Design review of the part built by this model. Coordinates are the model's own, in mm. Face numbers are marked on the shaded views. A direction names the side the tool comes from. Give positions to 0.01 mm unless a question says otherwise; leave off trailing zeros. Write each loop counter-clockwise with the first axis right and the second up, starting at its lowest first coordinate (ties: lowest second). Pieces come first, ordered by that corner, then holes.
```python
from build123d import *

# Parameters (mm, degrees)
F0_R     = 14.85
F0_R_2   = 2.25
F1_DEPTH = 13
F2_R     = 15.05
F3_DEPTH = 6
F4_R     = 14.6
F4_R_2   = 2.25
F5_DEPTH = 6.8
F6_R     = 2


with BuildPart() as f1:
    # F0 (on Top) → F1 (new body)
    with BuildSketch(Plane.XY):
        with BuildLine():
            ThreePointArc((10.083278, -13.5), (15.063627, -7.550472), (16.85, 0))
            ThreePointArc((16.85, 0), (15.063627, 7.550472), (10.083278, 13.5))
            ThreePointArc((10.083278, 13.5), (0, 16.85), (-10.083278, 13.5))
            ThreePointArc((-10.083278, 13.5), (-16.85, 0), (-10.083278, -13.5))
            ThreePointArc((-10.083278, -13.5), (0, -16.85), (10.083278, -13.5))
        make_face()
        Circle(F0_R, mode=Mode.SUBTRACT)
        with BuildLine():
            ThreePointArc((10.083278, 13.5), (15.063627, 7.550472), (16.85, 0))
            ThreePointArc((16.85, 0), (15.063627, -7.550472), (10.083278, -13.5))
            Line((10.083278, -13.5), (29.177113, -5.759277))
            ThreePointArc((29.177113, -5.759277), (30.538106, -4.655164), (31.05, -2.979058))
            Line((31.05, -2.979058), (31.05, 0))
            Line((31.05, 0), (31.05, 2.979058))
            ThreePointArc((31.05, 2.979058), (30.538106, 4.655164), (29.177113, 5.759277))
            Line((29.177113, 5.759277), (10.083278, 13.5))
        make_face()
        with Locations((24.05, 0)):
            Circle(F0_R_2, mode=Mode.SUBTRACT)
        with BuildLine():
            ThreePointArc((-10.083278, -13.5), (-16.85, 0), (-10.083278, 13.5))
            Line((-10.083278, 13.5), (-29.177113, 5.759277))
            ThreePointArc((-29.177113, 5.759277), (-30.538106, 4.655164), (-31.05, 2.979058))
            Line((-31.05, 2.979058), (-31.05, 0))
            Line((-31.05, 0), (-31.05, -2.979058))
            ThreePointArc((-31.05, -2.979058), (-30.538106, -4.655164), (-29.177113, -5.759277))
            Line((-29.177113, -5.759277), (-10.083278, -13.5))
        make_face()
        with Locations((-24.05, 0)):
            Circle(F0_R_2, mode=Mode.SUBTRACT)
    extrude(amount=F1_DEPTH)

    # F2 (on face) → F3 (join)
    with BuildSketch(Plane.XY.offset(13)):
        Circle(F2_R)
    extrude(amount=-F3_DEPTH)

    # F4 (on face) → F5 (join)
    with BuildSketch(Plane.XY.offset(13)):
        Circle(F4_R)
        Circle(F4_R_2, mode=Mode.SUBTRACT)
    extrude(amount=F5_DEPTH)

    # F6
    f6_edges = [f1.edges().sort_by_distance(p)[0] for p in [
        (-14.6, 0, 19.8),
    ]]
    fillet(f6_edges, radius=F6_R)


solid = f1.part
```
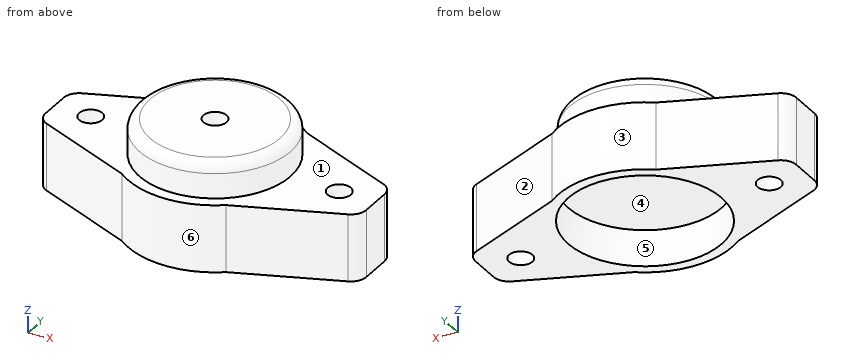
(1) Mouldability with a two-part tool opening along Y and no side actions: class the marked faces 3, 4, 5 and 6 as pulls with the +Y half, pulls with the -Y half, needs draft (parallel to the pull), parting line crosses it, or undercut.
Resolved:
face 3: pulls with the +Y half
face 4: undercut
face 5: undercut
face 6: pulls with the -Y half
(2) Consider section D-D, the plane z = 16.75. Give the boundary of the cut face in (x, y), then the cut area to 3 significant figures.
Resolved:
outline: circle Ø29.2 at (0, 0); hole circle Ø4.5 at (0, 0)
area: 654 mm2
(3) Consider section C-C, the plane x = 0. Give the boundary of the cut face in (y, z), then the cut area to 3 significant figures.
Resolved:
outline: (-16.85, 0) - (-14.85, 0) - (-14.85, 7) - (14.85, 7) - (14.85, 0) - (16.85, 0) - (16.85, 13) - (14.6, 13) - (14.6, 17.8) arc R2 ccw to (12.6, 19.8) - (2.25, 19.8) - (2.25, 13) - (-2.25, 13) - (-2.25, 19.8) - (-12.6, 19.8) arc R2 ccw to (-14.6, 17.8) - (-14.6, 13) - (-16.85, 13) - close
area: 396 mm2
(4) Tool access review of the marked faces 1 and 2: name each direction out of +Z, -Z, +X, -X, +Y, -Y from which nothing blocks a thin tool from reaching the whole face with its end or side.
Resolved:
face 1: +Z
face 2: +Z, -Z, +X, +Y
(5) Consider section B-B, the plane z = 3.75. Give the boundary of the cut face in (x, y).
Resolved:
outline: (-31.05, -2.98) arc R3 ccw to (-29.18, -5.76) - (-10.08, -13.5) arc R16.85 ccw to (10.08, -13.5) - (29.18, -5.76) arc R3 ccw to (31.05, -2.98) - (31.05, 2.98) arc R3 ccw to (29.18, 5.76) - (10.08, 13.5) arc R16.85 ccw to (-10.08, 13.5) - (-29.18, 5.76) arc R3 ccw to (-31.05, 2.98) - close; hole circle Ø4.5 at (-24.05, 0); hole circle Ø29.7 at (0, 0); hole circle Ø4.5 at (24.05, 0)
(6) Consider section A-A, the plane y = 0. Give the boundary of the cut face in (x, z).
Resolved:
outline: (-31.05, 0) - (-26.3, 0) - (-26.3, 13) - (-31.05, 13) - close; (-21.8, 0) - (-14.85, 0) - (-14.85, 7) - (14.85, 7) - (14.85, 0) - (21.8, 0) - (21.8, 13) - (14.6, 13) - (14.6, 17.8) arc R2 ccw to (12.6, 19.8) - (2.25, 19.8) - (2.25, 13) - (-2.25, 13) - (-2.25, 19.8) - (-12.6, 19.8) arc R2 ccw to (-14.6, 17.8) - (-14.6, 13) - (-21.8, 13) - close; (26.3, 0) - (31.05, 0) - (31.05, 13) - (26.3, 13) - close
(7) Clearance check with flat-ended pins moving along their axes: P1, Ø15, axis at x = 5, y = -2.5, coming from the -Z side; P2, Ø6, axis at x = 12, z = 14.5, coming from the +Y side; P3, Ø8, axis at x = 6.5, z = 9, coming from the +Y side. State where each tip first meets the part, or that it passes through.
Resolved:
P1: stops at z = 7
P2: stops at y = 13.98
P3: stops at y = 16.66
(8) To check wall thickness, follow L1, parallel to Y at x = 0, z = 2.75; L2, parallel to Z at x = 2, y = 6; L3, parallel to Z at x = -14, y = 10. State the ranges of each line that lie inside material, in increasing order.
Resolved:
L1: y = -16.85 to -14.85, 14.85 to 16.85
L2: z = 7 to 19.8
L3: z = 0 to 13
